from build123d import *

# Parameters (mm, degrees)
SKETCH2_R           = 76.2
SKETCH2_R_2         = 5
BOSS_EXTRUDE1_DEPTH = 15.875
CUT_EXTRUDE1_DEPTH  = 16.875
CIRPATTERN1_COUNT   = 32


with BuildPart() as part:
    # Sketch2 → Boss-Extrude1 (new body)
    with BuildSketch(Plane(origin=(0, 0, 0), x_dir=(1, 0, 0), z_dir=(0, 1, 0))):
        Circle(SKETCH2_R)
        Circle(SKETCH2_R_2, mode=Mode.SUBTRACT)
    extrude(amount=BOSS_EXTRUDE1_DEPTH)

    # Sketch3 → Cut-Extrude1 (cut, through all)
    with BuildSketch(Plane(origin=(0, 15.875, 0), x_dir=(1, 0, 0), z_dir=(0, 1, 0))):
        with BuildLine():
            Line((-4.264240487, 69.71971567), (-3.87658226, 63.3815597))
            ThreePointArc((-3.87658226, 63.3815597), (0, 63.5), (3.87658226, 63.3815597))
            Line((3.87658226, 63.3815597), (4.264240487, 69.71971567))
            ThreePointArc((4.264240487, 69.71971567), (0, 69.85), (-4.264240487, 69.71971567))
        make_face()
    cut_extrude1 = extrude(amount=-CUT_EXTRUDE1_DEPTH, mode=Mode.SUBTRACT)

    # CirPattern1: Cut-Extrude1 ×32 about axis
    cirpattern1_axis = Axis((0, 0, 0), (0, 1, 0))
    for i in range(1, CIRPATTERN1_COUNT):
        add(cut_extrude1.rotate(cirpattern1_axis, i * 360 / CIRPATTERN1_COUNT), mode=Mode.SUBTRACT)


solid = part.part
For this review, take the finished solid that the model builds, in its own axes (mm). Give positions to 0.01 mm unless a question says otherwise; leave off trailing zeros. Order: outer loops, then holes, each group sorted by start corner. A loop starts at its lowest first (then second) coordinate and runs counter-clockwise, first axis right, second up. Notation, with made-up numbers: (46.25, 88.25) -> (56.25, 88.25) arc R19 cw to (56.25, 113.25) -> close; hole circle Ø3 at (-12, 46). An arc over 180 degrees is marked (long way). Write item = value, one per line.
1) Insertion check: pin 1 (2 mm diameter, centred on x = 30, y = 3, fed in from -Z); pin 2 (5 mm diameter, centred on y = 12.5, z = -25, fed in from -X); pin 3 (1 mm diameter, centred on y = 9, z = -15.5, fed in from -X). Each pin has a flat end and moves straight along its axis. Give the tip position at first contact, or say it passes through.
Findings:
pin_1 = -70.47
pin_2 = -72.8
pin_3 = -74.71
2) To check wall thickness, follow L1, parallel to X at y = 11, z = 0; L2, parallel to Z at x = -53.5, y = 4. State the ranges of each line that lie inside material, in increasing order. Write a range as from..to.
Findings:
L1 = -76.2..-69.85, -63.5..-5, 5..63.5, 69.85..76.2
L2 = -54.26..-40.68, -34.21..34.21, 40.68..54.26
3) We need section B-B, the plane z = 0. Give the boundary of the cut face in (x, y) (3 decimals), and give its area (3 significant figures).
Findings:
outline = (-76.2, 0) -> (-69.85, 0) -> (-69.85, 15.875) -> (-76.2, 15.875) -> close; (-63.5, 0) -> (-5, 0) -> (-5, 15.875) -> (-63.5, 15.875) -> close; (5, 0) -> (63.5, 0) -> (63.5, 15.875) -> (5, 15.875) -> close; (69.85, 0) -> (76.2, 0) -> (76.2, 15.875) -> (69.85, 15.875) -> close
area = 2,060 mm^2
4) We need section C-C, the plane y = 8.5. Count the separate pieces of the cut face and the enclosed holes in it, and give its area (3 significant figures).
Findings:
separate_pieces = 1
enclosed_holes = 33
area = 16,500 mm^2
5) We need section A-A, the plane x = 0. Give the boundary of the cut face in (y, z) (3 decimals), and give its area (3 significant figures).
Findings:
outline = (0, -76.2) -> (15.875, -76.2) -> (15.875, -69.85) -> (0, -69.85) -> close; (0, -63.5) -> (15.875, -63.5) -> (15.875, -5) -> (0, -5) -> close; (0, 5) -> (15.875, 5) -> (15.875, 63.5) -> (0, 63.5) -> close; (0, 69.85) -> (15.875, 69.85) -> (15.875, 76.2) -> (0, 76.2) -> close
area = 2,060 mm^2
